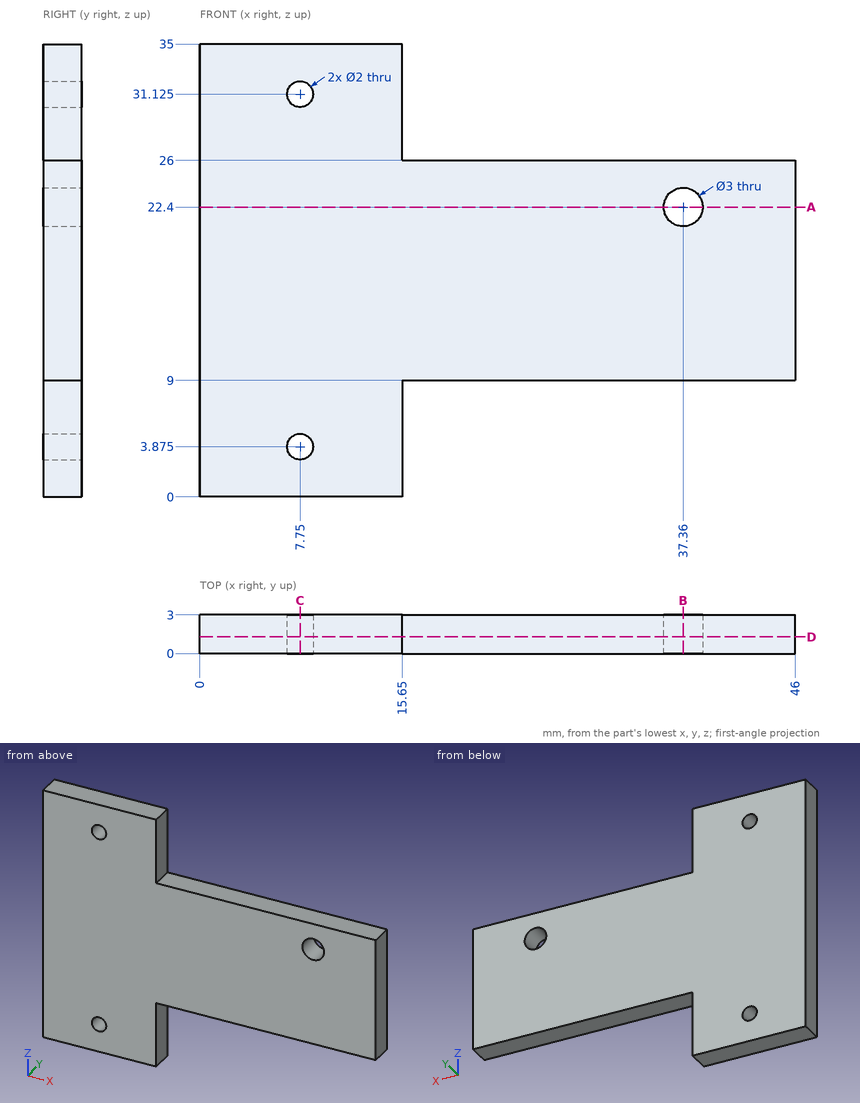
Here's the drawing with two shaded views (mm, measured from the low corner). I have some questions. Give positions to 0.01 mm unless a question says otherwise; leave off trailing zeros. Loops run counter-clockwise (first coordinate to the right, second up) from the corner with the lowest first, then second, coordinate; pieces in that order, holes last. Notation, with made-up numbers: (-1.75, 43) -> (55.25, 43) arc R26 cw to (55.25, 71) -> close; hole circle Ø2 at (-32.75, -32.5). An arc over 180 degrees is marked (long way). Use one line per item in the form item = value.
1) Will these pins go through, and if not, where does the flat tip stop? pin 1 (1.5 mm diameter, centred on y = 1.5, z = 29.5, fed in from +X); pin 2 (2.5 mm diameter, centred on x = 7.75, z = 3.875, fed in from -Y); pin 3 (1.5 mm diameter, centred on x = 28.5, y = 0.5, fed in from +Z).
Answers:
pin_1 = 15.65
pin_2 = 0
pin_3 = 26
2) I need wall thicknesses on line 1 along Z through (x, y) = (7.75, 1.65) (3 decimals); line 2 along Z through (x, y) = (37.36, 1.05); line 3 along Z through (x, y) = (21.5, 1.3). Which ranges of each line are inside material? Lowest first, please.
Answers:
line_1 = 0 to 2.875, 4.875 to 30.125, 32.125 to 35
line_2 = 9 to 20.9, 23.9 to 26
line_3 = 9 to 26
3) If we section it at C-C (x = 7.75): Please give me the cut outline in (y, z) (3 decimals).
Answers:
outline = (0, 0) -> (3, 0) -> (3, 2.875) -> (0, 2.875) -> close; (0, 4.875) -> (3, 4.875) -> (3, 30.125) -> (0, 30.125) -> close; (0, 32.125) -> (3, 32.125) -> (3, 35) -> (0, 35) -> close
4) If we section it at D-D (y = 1.3): Please give me the cut outline in (x, z) (3 decimals), plus the area to 3 significant figures.
Answers:
outline = (0, 0) -> (15.65, 0) -> (15.65, 9) -> (46, 9) -> (46, 26) -> (15.65, 26) -> (15.65, 35) -> (0, 35) -> close; hole circle Ø2 at (7.75, 3.875); hole circle Ø2 at (7.75, 31.125); hole circle Ø3 at (37.36, 22.4)
area = 1,050 mm²
5) If we section it at A-A (z = 22.4): Please give me the cut outline in (x, y).
Answers:
outline = (0, 0) -> (35.86, 0) -> (35.86, 3) -> (0, 3) -> close; (38.86, 0) -> (46, 0) -> (46, 3) -> (38.86, 3) -> close
6) If we section it at B-B (x = 37.36): Please give me the cut outline in (y, z).
Answers:
outline = (0, 9) -> (3, 9) -> (3, 20.9) -> (0, 20.9) -> close; (0, 23.9) -> (3, 23.9) -> (3, 26) -> (0, 26) -> close
